Can you work these out from the drawing? Everything is in mm from the part's minimum corner. Round coordinates to 2 decimals unless told otherwise and drop trailing zeros. Order: outer loops, then holes, each group sorted by start corner. A loop starts at its lowest first (then second) coordinate and runs counter-clockwise, first axis right, second up. Notation, with made-up numbers: (36.5, 57) - (69.5, 57) arc R21 ccw to (69.5, 66) - close; hole circle Ø9 at (56.5, 52). An arc over 180 degrees is marked (long way). Write item = value, one per line.
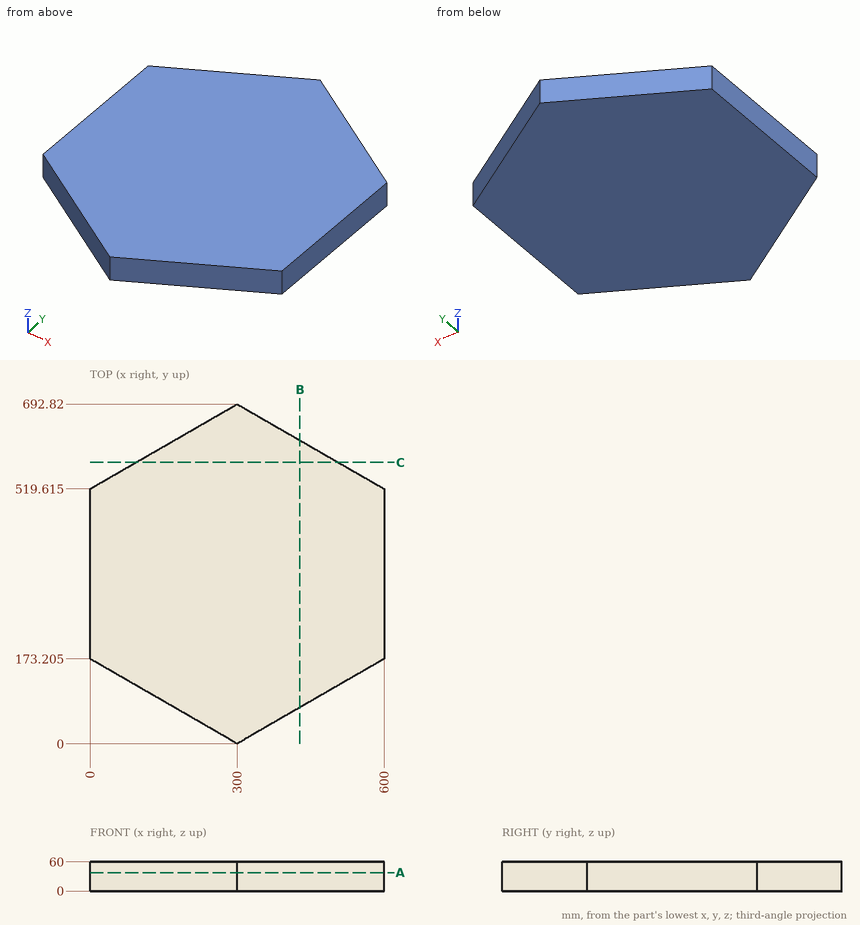
(1) If we section it at C-C (y = 574): Write out the boundary of the cut face in (x, z).
Computed:
outline = (94.2, 0) - (505.8, 0) - (505.8, 60) - (94.2, 60) - close
(2) Will these pins go through, and if not, where does the flat tip stop? P1, Ø6, axis at x = 486.5, z = 21.5, coming from the -Y side; P2, Ø8, axis at x = 84.5, z = 46.5, coming from the +Y side; P3, Ø6, axis at x = 240.5, z = 33.5, coming from the -Y side.
Computed:
P1 = 105.94
P2 = 570.71
P3 = 32.62
(3) If we section it at B-B (x = 428): Write out the boundary of the cut face in (y, z), plus the area to 3 significant figures.
Computed:
outline = (73.9, 0) - (618.92, 0) - (618.92, 60) - (73.9, 60) - close
area = 32,700 mm^2
(4) If I drill on line 1 (X direction, y = 573.5, z = 12); line 2 (Y direction, x = 178, z = 6) (1 decimal); line 3 (X direction, y = 156, z = 22), over which ranges is the centre line in solid material (lowest first)? Write a range as from..to.
Computed:
line_1 = 93.33..506.67
line_2 = 70.4..622.4
line_3 = 29.8..570.2
(5) If we section it at A-A (z = 38): Write out the boundary of the cut face in (x, y) (1 decimal).
Computed:
outline = (0, 173.2) - (300, 0) - (600, 173.2) - (600, 519.6) - (300, 692.8) - (0, 519.6) - close
